```python
from build123d import *

# Parameters (mm, degrees)
F0_R     = 25.065
F1_DEPTH = 38.13
F2_R     = 20.75
F3_DEPTH = 20.3
F5_R     = 5


# Not quite as in the source:
# - a fillet or chamfer that OpenCascade refuses, or shapes differently, is made with other operations: its cross-section is extruded or revolved along the edge and cut away or added


with BuildPart() as f1:
    # F0 (on Top) → F1 (new body, symmetric)
    with BuildSketch(Plane.XY):
        Circle(F0_R)
    extrude(amount=F1_DEPTH, both=True)

    # F2 (on face) → F3 (join)
    with BuildSketch(Plane.XY.offset(38.13)):
        Circle(F2_R)
    extrude(amount=F3_DEPTH)

    # F4: fillet of radius 7 on 2 edges, made by hand

    # F4_s1 → F4_t2 (revolve, cut)
    with BuildSketch(Plane.XZ):
        with BuildLine():
            ThreePointArc((25.065, 31.6654215141), (23.8871559581, 35.5516150245), (20.75, 38.13))
            Line((20.75, 38.13), (25.065, 38.13))
            Line((25.065, 38.13), (25.065, 31.6654215141))
        make_face()
    revolve(axis=Axis((0, 0, 38.13), (0, 0, 1)), mode=Mode.SUBTRACT)

    # F4_s3 → F4_t4 (revolve, cut)
    with BuildSketch(Plane.XZ):
        with BuildLine():
            ThreePointArc((25.065, -31.13), (23.0147474683, -36.0797474683), (18.065, -38.13))
            Line((18.065, -38.13), (25.065, -38.13))
            Line((25.065, -38.13), (25.065, -31.13))
        make_face()
    revolve(axis=Axis((0, 0, -38.13), (0, 0, 1)), mode=Mode.SUBTRACT)

    # F5
    f5_edges = [f1.edges().sort_by_distance(p)[0] for p in [
        (-20.75, 0, 58.43),
    ]]
    fillet(f5_edges, radius=F5_R)


solid = f1.part
```
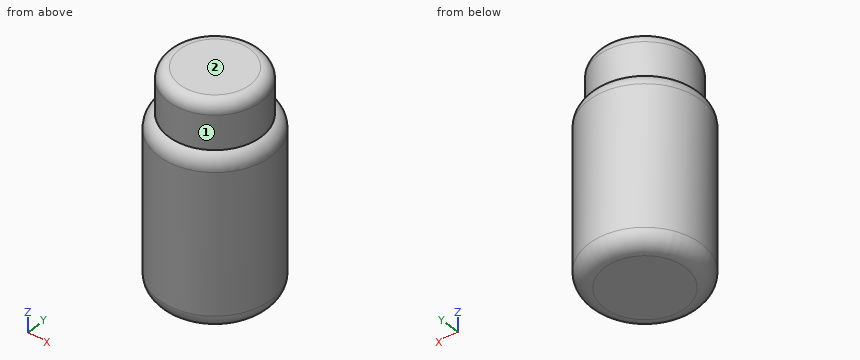
Input: part model. Units: mm. Frame: model coordinates. Face numbers are marked on the shaded views. A direction names the side the tool comes from. Coordinates: 2 decimals unless noted, no trailing zeros. Write each loop counter-clockwise with the first axis right and the second up, starting at its lowest first coordinate (ties: lowest second). Pieces come first, ordered by that corner, then holes. Notation, with made-up numbers: (-31, -34) -> (-15, -34) arc R23 ccw to (-15, 4) -> close; hole circle Ø3 at (87, -8). An arc over 180 degrees is marked (long way). Answer as a JSON object with one key per item and string values.
1. First-contact query: P1, Ø3, axis at y = -18, z = 1, coming from the +X side; P2, Ø1, axis at x = -6, z = 43, coming from the +Y side; P3, Ø8, axis at y = -3, z = -25.5, coming from the -X side (3 decimals); P4, Ø1.5, axis at y = -1.5, z = 44.5, coming from the +X side. Flat tips, straight axial feed; report the tip coordinate or a pass-through.
Result set:
{"P1": "stops at x = 18.87", "P2": "stops at y = 20.01", "P3": "stops at x = -25.065", "P4": "stops at x = 20.74"}
2. Material intervals for line 1 (X direction, y = 0.5, z = -19.5); line 2 (Y direction, x = -19, z = -9.5); line 3 (Z direction, x = 18, y = -0.5), sorted ascending. Write a range as from..to.
Result set:
{"line 1": "x = -25.06..25.06", "line 2": "y = -16.35..16.35", "line 3": "z = -38.13..57.89"}
3. Section A-A on y = 0. Return the cut outline in (x, z) (3 decimals), then the cut area to 3 significant figures.
Result set:
{"outline": "(-25.065, -31.13) arc R7 ccw to (-18.065, -38.13) -> (18.065, -38.13) arc R7 ccw to (25.065, -31.13) -> (25.065, 31.665) arc R7 ccw to (20.75, 38.13) -> (20.75, 53.43) arc R5 ccw to (15.75, 58.43) -> (-15.75, 58.43) arc R5 ccw to (-20.75, 53.43) -> (-20.75, 38.13) arc R7 ccw to (-25.065, 31.665) -> close", "area": "4,620 mm2"}
4. Section C-C on z = -5. Return the cut outline in (x, y) (3 decimals).
Result set:
{"outline": "circle Ø50.13 at (0, 0)"}
5. Access query for the marked faces 1 and 2. Directions: +Z, -Z, +X, -X, +Y, -Y. A direction counts if a zero-diameter tool reaches every point of the face in a straight line with its end or side. Return the directions, or none.
Result set:
{"face 1": "+Z", "face 2": "+Z, +X, -X, +Y, -Y"}
